Could you check a few things on this model? Use its own coordinates, in mm. Face numbers are marked on the shaded views. A direction names the side the tool comes from. Give positions to 0.01 mm unless a question says otherwise; leave off trailing zeros. Order: outer loops, then holes, each group sorted by start corner. A loop starts at its lowest first (then second) coordinate and runs counter-clockwise, first axis right, second up. Notation, with made-up numbers: (28, -37) -> (44, -37) arc R26 cw to (44, 1) -> close; hole circle Ø4 at (-34, 78). An arc over 180 degrees is marked (long way). Use one line per item in the form item = value. Start each with the question number.
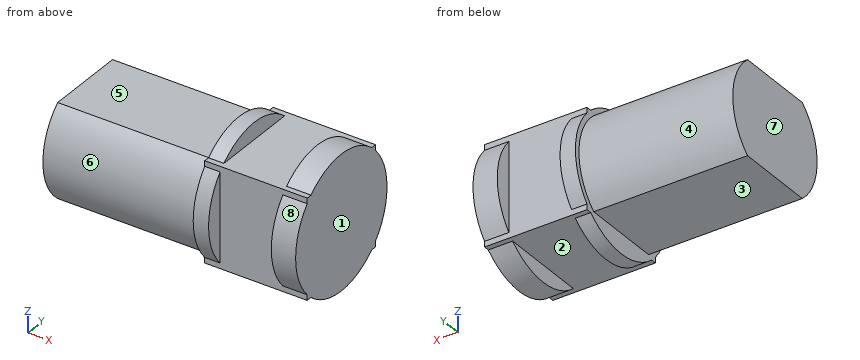
from build123d import *

# Parameters (mm, degrees)
SKETCH1_W           = 16.51
SKETCH1_H           = 16.51
BOSS_EXTRUDE1_DEPTH = 8.4582
SKETCH2_R           = 11.049
BOSS_EXTRUDE2_DEPTH = 4.0132
BOSS_EXTRUDE3_START = -2.54
SKETCH3_R           = 11.049
BOSS_EXTRUDE3_DEPTH = 2.54
BOSS_EXTRUDE4_DEPTH = 25.4


with BuildPart() as part:
    # Sketch1 → Boss-Extrude1 (new, symmetric)
    with BuildSketch(Plane(origin=(0, 0, 0), x_dir=(0, 0, -1), z_dir=(1, 0, 0))):
        Rectangle(SKETCH1_W, SKETCH1_H)
    extrude(amount=BOSS_EXTRUDE1_DEPTH, both=True)

    # Sketch2 → Boss-Extrude2 (add)
    with BuildSketch(Plane(origin=(8.4582, 0, 0), x_dir=(0, 0, -1), z_dir=(1, 0, 0))):
        Circle(SKETCH2_R)
    extrude(amount=-BOSS_EXTRUDE2_DEPTH)

    # Sketch3 → Boss-Extrude3 (add)
    with BuildSketch(Plane.ZY.offset(8.4582).offset(BOSS_EXTRUDE3_START)):
        Circle(SKETCH3_R)
    extrude(amount=BOSS_EXTRUDE3_DEPTH)

    # Sketch4 → Boss-Extrude4 (add)
    with BuildSketch(Plane.ZY.offset(8.4582)):
        with BuildLine():
            Line((-7.747, -6.632136504), (-7.747, 6.632136504))
            ThreePointArc((-7.747, 6.632136504), (0, 10.1981), (7.747, 6.632136504))
            Line((7.747, 6.632136504), (7.747, -6.632136504))
            ThreePointArc((7.747, -6.632136504), (0, -10.1981), (-7.747, -6.632136504))
        make_face()
    extrude(amount=BOSS_EXTRUDE4_DEPTH)


solid = part.part
(1) Which directions (+Z, -Z, +X, -X, +Y, -Y) give clear straight access to the entire face, cutting with the end or side of a thin tool? Please do the marked faces 4, 5, 6, 7 and 8.
(2) We'd pull the mould along X, two halves only. Please class the marked faces 1, 2 and 3: pulls with the +X half, pulls with the -X half, needs draft (parallel to the pull), parting line crosses it, or undercut.
(3) I'm going to push flat-ended pins straight in: pin 1 Ø12 at (x, z) = (-23.5, 4.5) entering from +Y; pin 2 Ø6 at (x, z) = (-22, 6) entering from -Y; pin 3 Ø8.5 at (x, y) = (0, -3) entering from -Z (3 decimals). Where does each tip first touch, or does it pass through?
(4) Imagine slicing it at B-B (z = 8.75). Write out the boundary of the cut face in (x, y) (3 decimals).
(5) Imagine slicing it at A-A (y = 9.5). Write out the boundary of the cut face in (x, z) (3 decimals).
(6) Please list where these lines run through material, in increasing order: probe 1 along X at (y, z) = (-8.5, -4.25) (3 decimals); probe 2 along X at (y, z) = (2.5, 9.75) (3 decimals); probe 3 along Z at (x, y) = (-22, 0.5).
(7) Imagine slicing it at D-D (y = 1.75). Write out the boundary of the cut face in (x, z) (3 decimals), plus the area to 3 significant figures.
(8) Imagine slicing it at C-C (x = -27.5). Write out the boundary of the cut face in (y, z).
Calculated:
q1.face_4 = -X, +Y
q1.face_5 = +Z, -X, +Y, -Y
q1.face_6 = -X, -Y
q1.face_7 = +Z, -Z, -X, +Y, -Y
q1.face_8 = +X, -X, -Y
q2.face_1 = pulls with the +X half
q2.face_2 = undercut
q2.face_3 = needs draft
q3.pin_1 = 10.2
q3.pin_2 = -9.75
q3.pin_3 = -8.255
q4.outline = (-8.458, -6.747) -> (-5.918, -6.747) -> (-5.918, 6.747) -> (-8.458, 6.747) -> close; (4.445, -6.747) -> (8.458, -6.747) -> (8.458, 6.747) -> (4.445, 6.747) -> close
q5.outline = (-33.858, -3.708) -> (-8.458, -3.708) -> (-8.458, -5.642) -> (-5.918, -5.642) -> (-5.918, 5.642) -> (-8.458, 5.642) -> (-8.458, 3.708) -> (-33.858, 3.708) -> close; (4.445, -5.642) -> (8.458, -5.642) -> (8.458, 5.642) -> (4.445, 5.642) -> close
q6.probe_1 = -33.858 to -5.918, 4.445 to 8.458
q6.probe_2 = -8.458 to -5.918, 4.445 to 8.458
q6.probe_3 = -7.75 to 7.75
q7.outline = (-33.858, -7.747) -> (-8.458, -7.747) -> (-8.458, -10.91) -> (-5.918, -10.91) -> (-5.918, -8.255) -> (4.445, -8.255) -> (4.445, -10.91) -> (8.458, -10.91) -> (8.458, 10.91) -> (4.445, 10.91) -> (4.445, 8.255) -> (-5.918, 8.255) -> (-5.918, 10.91) -> (-8.458, 10.91) -> (-8.458, 7.747) -> (-33.858, 7.747) -> close
q7.area = 708 mm2
q8.outline = (-6.63, -7.75) -> (6.63, -7.75) arc R10.2 ccw to (6.63, 7.75) -> (-6.63, 7.75) arc R10.2 ccw to start
